from build123d import *

# Parameters (mm, degrees)
SKETCH1_W                  = 63.5
SKETCH1_H                  = 88.9
BOSS_EXTRUDE1_DEPTH        = 18.13868
CUT_EXTRUDE1_DEPTH         = 63.5
SKETCH5_W                  = 1.7272
SKETCH5_H                  = 8.613680223
F_8_0_199_DIAMETER_HOLE1_D = 5.0546


with BuildPart() as part:
    # Sketch1 → Boss-Extrude1 (new body)
    with BuildSketch(Plane.XY):
        with Locations((-78.907526017, 47.538989794)):
            Rectangle(SKETCH1_W, SKETCH1_H)
    extrude(amount=BOSS_EXTRUDE1_DEPTH)

    # Sketch2 → Cut-Extrude1 (cut)
    with BuildSketch(Plane.ZY.offset(110.657526017)):
        with BuildLine():
            Line((8.613680223, 91.988989794), (8.613680223, 74.018491939))
            Line((8.613680223, 74.018491939), (8.613680223, 69.243291939))
            Line((8.613680223, 69.243291939), (8.613680223, 68.805550488))
            ThreePointArc((8.613680223, 68.805550488), (8.619201776, 68.494519524), (8.635759479, 68.183880521))
            ThreePointArc((8.635759479, 68.183880521), (9.666013904, 64.641922993), (12.0625652, 61.83774233))
            Line((12.0625652, 61.83774233), (13.078006955, 61.063298751))
            Line((13.078006955, 61.063298751), (13.67435349, 60.608485127))
            Line((13.67435349, 60.608485127), (14.689795245, 59.834041549))
            ThreePointArc((14.689795245, 59.834041549), (17.086346542, 57.029860886), (18.116600967, 53.487903358))
            ThreePointArc((18.116600967, 53.487903358), (18.133158669, 53.177264354), (18.138680223, 52.866233391))
            Line((18.138680223, 52.866233391), (18.138680223, 91.988989794))
            Line((18.138680223, 91.988989794), (8.613680223, 91.988989794))
        make_face()
    extrude(amount=-CUT_EXTRUDE1_DEPTH, mode=Mode.SUBTRACT)

    # Sketch5 → #29 (0.136) Diameter Hole1 (revolve, cut)
    with BuildSketch(Plane(origin=(-80.764740239, 69.243291939, 8.613680223), x_dir=(0, -1, 0), z_dir=(1, 0, 0))):
        with Locations((0.8636, 4.306840112)):
            Rectangle(SKETCH5_W, SKETCH5_H)
    revolve(axis=Axis((-80.764740239, 69.243291939, 14.963680223), (0, 0, -1)), mode=Mode.SUBTRACT)

    # #8 (0.199) Diameter Hole1 (through all)
    with Locations(Plane.XY.offset(18.138680223)):
        with Locations((-80.777440239, 14.315791939)):
            Hole(F_8_0_199_DIAMETER_HOLE1_D / 2)


solid = part.part
Read the model definition and answer for the solid it produces. Units are mm, in the model's axes. A direction names the side the tool comes from. Coordinates: 2 decimals unless noted, no trailing zeros. Loops run counter-clockwise (first coordinate to the right, second up) from the corner with the lowest first, then second, coordinate; pieces in that order, holes last. Notation, with made-up numbers: (4, 14) - (55, 14) arc R17 ccw to (55, 45) - close; hole circle Ø6 at (4, 69). An arc over 180 degrees is marked (long way). Answer in a Markdown table with one row per item.
Q1. Straight lines are drawn through the part: line 1 along Z through (x, y) = (-72, 75.5); line 2 along Z through (x, y) = (-57, 54); line 3 along Y through (x, z) = (-57, 17.25). For each, find the intervals that lie inside material, in ascending order. Write a range as [from, to].
Here are the results:
| item | result |
|---|---|
| line 1 | z = [0, 8.61] |
| line 2 | z = [0, 18.07] |
| line 3 | y = [3.09, 56.71] |
Q2. Find section C-C on z = 10.75. Write down the section's boundary in (x, y).
Here are the results:
| item | result |
|---|---|
| outline | (-110.66, 3.09) - (-47.16, 3.09) - (-47.16, 63.07) - (-110.66, 63.07) - close; hole circle Ø5.05 at (-80.78, 14.32) |
Q3. Find section A-A on x = -85. Write down the section's boundary in (y, z), plus the area to 3 significant figures.
Here are the results:
| item | result |
|---|---|
| outline | (3.09, 0) - (91.99, 0) - (91.99, 8.61) - (68.81, 8.61) arc R8.76 cw to (61.84, 12.06) - (59.83, 14.69) arc R8.76 ccw to (52.87, 18.14) - (3.09, 18.14) - close |
| area | 1,320 mm^2 |
Q4. For faces 4 (the flat face through (-79, 81, 8.614)), 5 (the flat face through (-79, 48, 0)), determine the directions among +Z, -Z, +X, -X, +Y, -Y from which every point of the face is accessible in a straight line to the end or side of a thin tool.
Here are the results:
| item | result |
|---|---|
| face 4 | +Z, +X, -X, +Y |
| face 5 | -Z, +X, -X, +Y, -Y |
Q5. Given P1, Ø4, axis at x = -70, z = 12, coming from the +Y side, flat-ended and moving along its own axis, determine where the tip first touches the part or whether it passes through.
Here are the results:
| item | result |
|---|---|
| P1 | stops at y = 64.08 |
Q6. The mould has two halves that part along X. Classify faces 1 (the cylindrical face through (-79.08, 69.62, 4.25)), 2 (the flat face through (-79, 91.989, 4)), 3 (the flat face through (-47.158, 37, 9)): pulls with the +X half, pulls with the -X half, needs draft (parallel to the pull), parting line crosses it, or undercut.
Here are the results:
| item | result |
|---|---|
| face 1 | undercut |
| face 2 | needs draft |
| face 3 | pulls with the +X half |
Q7. Find section B-B on y = 85. Write down the section's boundary in (x, z).
Here are the results:
| item | result |
|---|---|
| outline | (-110.66, 0) - (-47.16, 0) - (-47.16, 8.61) - (-110.66, 8.61) - close |
Q8. Find section D-D on y = 64.5. Write down the section's boundary in (x, z), plus the area to 3 significant figures.
Here are the results:
| item | result |
|---|---|
| outline | (-110.66, 0) - (-47.16, 0) - (-47.16, 9.74) - (-110.66, 9.74) - close |
| area | 619 mm^2 |
